Work out the finished part from the listing and answer in its coordinate system (mm). A direction names the side the tool comes from. Coordinates: 2 decimals unless noted, no trailing zeros. Write each loop counter-clockwise with the first axis right and the second up, starting at its lowest first coordinate (ties: lowest second). Pieces come first, ordered by that corner, then holes. Notation, with made-up numbers: (31.5, -36) - (72.5, -36) arc R11 cw to (72.5, -28) - close; hole circle Ø11 at (70, 45). An arc over 180 degrees is marked (long way). Answer as a JSON object with one key per item and string values. Group by question number.
from build123d import *

# Parameters (mm, degrees)
SKETCH2_R           = 7
BOSS_EXTRUDE1_DEPTH = 45


with BuildPart() as part:
    # Sketch2 → Boss-Extrude1 (new body)
    with BuildSketch(Plane.XY):
        with BuildLine():
            Line((-14, 11), (-14, -7))
            Line((-14, -7), (-7, -14))
            Line((-7, -14), (21.680626854, -14))
            ThreePointArc((21.680626854, -14), (25.029243776, -15.286946714), (26.654064081, -18.485294118))
            ThreePointArc((26.654064081, -18.485294118), (28.520286549, -26.134616219), (32.37533784, -33))
            Line((32.37533784, -33), (41, -33))
            Line((41, -33), (70, 2))
            Line((70, 2), (70, 21))
            Line((70, 21), (65, 26))
            Line((65, 26), (36, 26))
            ThreePointArc((36, 26), (27.554449431, 17.143424137), (15.460180615, 15.273953031))
            Line((15.460180615, 15.273953031), (0, 18))
            Line((0, 18), (-7, 18))
            Line((-7, 18), (-14, 11))
        make_face()
        Circle(SKETCH2_R, mode=Mode.SUBTRACT)
    extrude(amount=BOSS_EXTRUDE1_DEPTH)


solid = part.part
Q1. For a pull along Y with two mould halves and no side action, classify faces 1 (the face through (6.466, -2.681, 22.185)), 2 (the face through (28.48, -26.03, 22.18)), 3 (the face through (68, 23, 22)) as +Y half, -Y half, draft (parallel to the pull), parting line (faces both ways), or undercut.
Q2. Section D-D on x = 52.5 is taken. Determine the outline of the cut face in (y, z), plus the area to 3 significant figures.
Q3. Section B-B on y = 0 is taken. Determine the outline of the cut face in (x, z).
Q4. Section C-C on y = 6 is taken. Determine the outline of the cut face in (x, z), plus the area to 3 significant figures.
Q5. Flat-ended cylindrical pins translate along their axes: pin 1 Ø5.5 at (x, z) = (-3.5, 11.5) entering from +Y; pin 2 Ø23 at (x, z) = (2, 14) entering from -Y; pin 3 Ø2 at (y, z) = (-16.5, 15.5) entering from -X. Find the tip coordinate at first contact, or state that the pin passes through.
Q6. Consider L1, parallel to Y at x = 0, z = 25; L2, parallel to X at y = 4.5, z = 30; L3, parallel to X at y = -2, z = 22. Determine where each line is inside the solid, lowest interval first. Write a range as from..to.
Q7. A tool of negligible diameter and unlimited length cuts with its end or side. For faces 4 (the face through (-3, 18, 22)), 5 (the face through (7, -14, 22)), 6 (the face through (37, 3, 0)), 7 (the face through (7.838, 16.618, 22.185)), from which of +Z, -Z, +X, -X, +Y, -Y can it reach the whole face along a straight path? Write none if from no direction.
Q8. Section A-A on z = 9 is taken. Determine the outline of the cut face in (x, y), plus the area to 3 significant figures.
Numbers:
{
 "1": {"face 1": "undercut", "face 2": "-Y half", "face 3": "+Y half"},
 "2": {"outline": "(-19.12, 0) - (26, 0) - (26, 45) - (-19.12, 45) - close", "area": "2,030 mm²"},
 "3": {"outline": "(-14, 0) - (-7, 0) - (-7, 45) - (-14, 45) - close; (7, 0) - (68.34, 0) - (68.34, 45) - (7, 45) - close"},
 "4": {"outline": "(-14, 0) - (-3.61, 0) - (-3.61, 45) - (-14, 45) - close; (3.61, 0) - (70, 0) - (70, 45) - (3.61, 45) - close", "area": "3,460 mm²"},
 "5": {"pin 1": "stops at y = 18", "pin 2": "stops at y = -14", "pin 3": "stops at x = 25.25"},
 "6": {"L1": "y = -14..-7, 7..18", "L2": "x = -14..-5.36, 5.36..70", "L3": "x = -14..-6.71, 6.71..66.69"},
 "7": {"face 4": "+Z, -Z, -X, +Y", "face 5": "+Z, -Z, -X, -Y", "face 6": "-Z, +X, -X, +Y, -Y", "face 7": "+Z, -Z, +Y"},
 "8": {"outline": "(-14, -7) - (-7, -14) - (21.68, -14) arc R5 cw to (26.65, -18.49) arc R29 ccw to (32.38, -33) - (41, -33) - (70, 2) - (70, 21) - (65, 26) - (36, 26) arc R19 cw to (15.46, 15.27) - (0, 18) - (-7, 18) - (-14, 11) - close; hole circle Ø14 at (0, 0)", "area": "3,010 mm²"}
}
